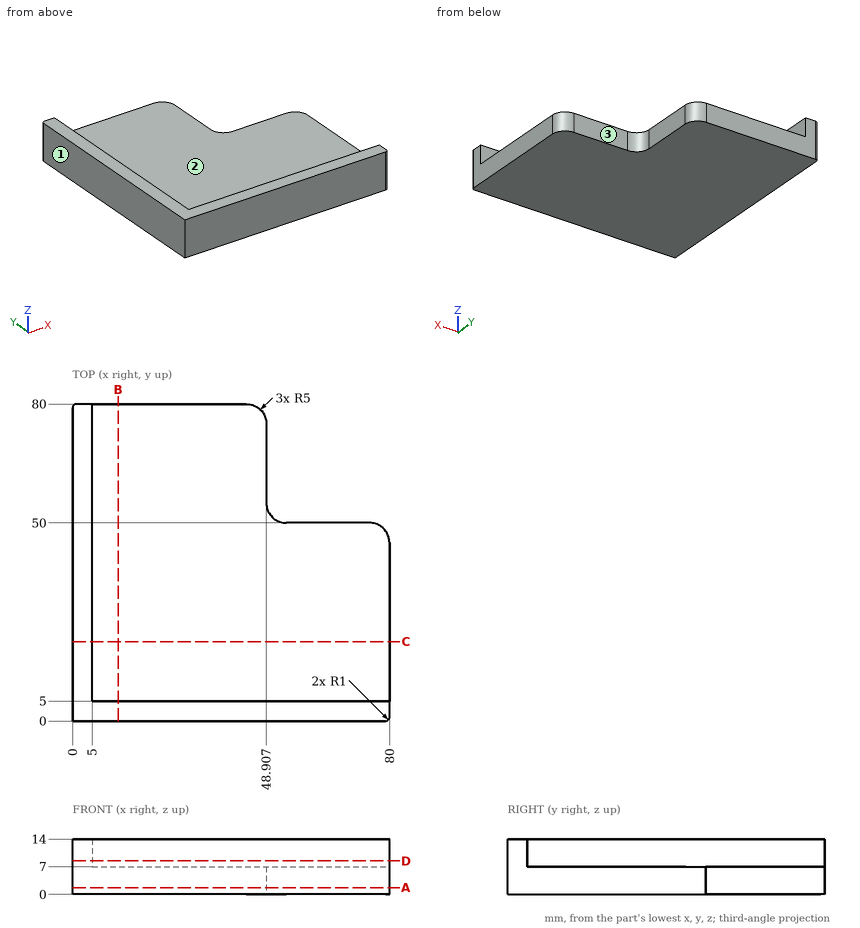
Design review of the part shown in the three views and the two pictorial views. Dimensions are in mm from the part's minimum x, y and z. A direction names the side the tool comes from. Round coordinates to 2 decimals unless told otherwise and drop trailing zeros. Loops run counter-clockwise (first coordinate to the right, second up) from the corner with the lowest first, then second, coordinate; pieces in that order, holes last. Notation, with made-up numbers: M -34.75,35 L -11.75,35 A11 cw -11.75,55 Z; hole C 2,-31 d8. An arc over 180 degrees is marked long. Answer as a JSON object with one key per item and string values.
Item 1: Wall thickness on L1, parallel to Z at x = 18, y = 70; L2, parallel to X at y = 43.5, z = 11; L3, parallel to Y at x = 54, z = 1.25: over which ranges is each line inside the solid? List them lowest first. Write a range as from..to.
Answer sheet:
{"L1": "z = 0..7", "L2": "x = 0..5", "L3": "y = 0..50"}
Item 2: We need section D-D on z = 8.5. Give the boundary of the cut face in (x, y).
Answer sheet:
{"outline": "M 0,0 L 79,0 A1 ccw 80,1 L 80,5 L 5,5 L 5,80 L 1,80 A1 ccw 0,79 Z"}
Item 3: We need section B-B on x = 11.5. Give the boundary of the cut face in (y, z).
Answer sheet:
{"outline": "M 0,0 L 80,0 L 80,7 L 5,7 L 5,14 L 0,14 Z"}
Item 4: We need section A-A on z = 1.75. Give the boundary of the cut face in (x, y), and give its area (3 significant figures).
Answer sheet:
{"outline": "M 0,0 L 79,0 A1 ccw 80,1 L 80,45 A5 ccw 75,50 L 53.91,50 A5 cw 48.91,55 L 48.91,75 A5 ccw 43.91,80 L 1,80 A1 ccw 0,79 Z", "area": "5,460 mm^2"}
Item 5: Machinability: for the marked faces 1, 2 and 3, which of the approach directions +Z, -Z, +X, -X, +Y, -Y give a long, thin tool a straight path to every point of the face, cutting with its end or side? Answer none if there is none.
Answer sheet:
{"face 1": "+Z, -Z, -X, +Y, -Y", "face 2": "+Z, +X, +Y", "face 3": "+Z, -Z, +X, +Y"}
Item 6: Clearance check with flat-ended pins moving along their axes: P1, Ø8, axis at x = 38, z = 12.5, coming from the +Y side; P2, Ø3.5, axis at y = 60, z = 2, coming from the +X side; P3, Ø5.5, axis at y = 56.5, z = 11, coming from the +X side; P4, Ø3, axis at x = 67.5, y = 22.5, coming from the -Z side. State where each tip first meets the part, or that it passes through.
Answer sheet:
{"P1": "stops at y = 5", "P2": "stops at x = 48.91", "P3": "stops at x = 5", "P4": "stops at z = 0"}
